Read the model definition and answer for the solid it produces. Units are mm, in the model's axes. Coordinates: 2 decimals unless noted, no trailing zeros. Order: outer loops, then holes, each group sorted by start corner. A loop starts at its lowest first (then second) coordinate and runs counter-clockwise, first axis right, second up. Notation, with made-up numbers: M 78.5,89 L 137.5,89 A25 cw 137.5,103 Z; hole C 69,-24 d11. An arc over 180 degrees is marked long. Write each question's results on one line, items separated by ' | '.
```python
from build123d import *

# Parameters (mm, degrees)
SKETCH12_R                   = 30.1625
SKETCH12_R_2                 = 26.2509
PIPE_STANDARD_S40_P2_1_DEPTH = 660.4
CUT_EXTRUDE1_DEPTH           = 662.7761803
CUT_EXTRUDE1_DEPTH_BACK      = 662.7761803
CUT_EXTRUDE2_DEPTH           = 662.7761803
CUT_EXTRUDE2_DEPTH_BACK      = 662.7761803
CUT_EXTRUDE3_DEPTH           = 662.7761803
CUT_EXTRUDE3_DEPTH_BACK      = 662.7761803


with BuildPart() as part:
    # Sketch12 → Pipe (standard, s40) P2(1) (new body)
    with BuildSketch(Plane(origin=(0, 0, 0), x_dir=(-1, 0, 0), z_dir=(0, 0, -1))):
        Circle(SKETCH12_R)
        Circle(SKETCH12_R_2, mode=Mode.SUBTRACT)
    extrude(amount=PIPE_STANDARD_S40_P2_1_DEPTH)

    # Sketch14 → Cut-Extrude1 (cut, two sides)
    with BuildSketch(Plane(origin=(0, 0, 0), x_dir=(1, 0, 0), z_dir=(0, 1, 0))) as cut_extrude1_sk:
        Polygon((0, 12.7), (-12.7, 0), (12.7, 0), align=None)
    extrude(amount=CUT_EXTRUDE1_DEPTH, mode=Mode.SUBTRACT)
    extrude(cut_extrude1_sk.sketch, amount=-CUT_EXTRUDE1_DEPTH_BACK, mode=Mode.SUBTRACT)

    # Sketch15 → Cut-Extrude2 (cut, two sides)
    with BuildSketch(Plane(origin=(0, 0, 0), x_dir=(0, 0, -1), z_dir=(0.8660254037844364, -0.5000000000000041, 0))) as cut_extrude2_sk:
        Polygon((0, 12.7), (0, -12.7), (12.7, 0), align=None)
    extrude(amount=CUT_EXTRUDE2_DEPTH, mode=Mode.SUBTRACT)
    extrude(cut_extrude2_sk.sketch, amount=-CUT_EXTRUDE2_DEPTH_BACK, mode=Mode.SUBTRACT)

    # Sketch16 → Cut-Extrude3 (cut, two sides)
    with BuildSketch(Plane(origin=(0, 0, 0), x_dir=(0, 0, -1), z_dir=(-0.8660254037844433, -0.49999999999999195, 0))) as cut_extrude3_sk:
        Polygon((0, 12.7), (0, -12.7), (12.7, 0), align=None)
    extrude(amount=CUT_EXTRUDE3_DEPTH, mode=Mode.SUBTRACT)
    extrude(cut_extrude3_sk.sketch, amount=-CUT_EXTRUDE3_DEPTH_BACK, mode=Mode.SUBTRACT)


solid = part.part
```
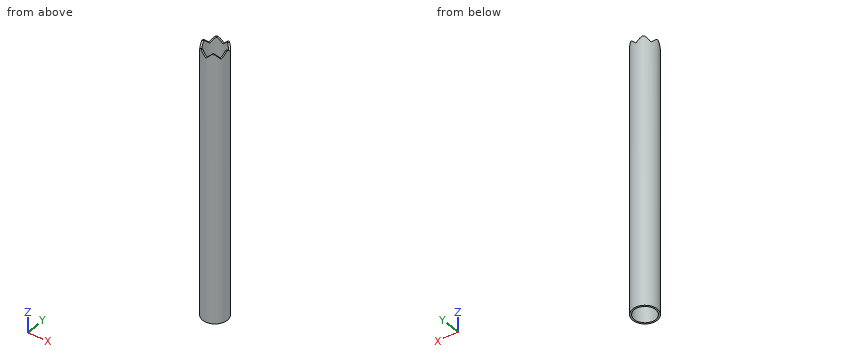
(1) Straight lines are drawn through the part: line 1 (Y direction, x = 0, z = -319); line 2 (Y direction, x = -22, z = -120.5); line 3 (X direction, y = -9.5, z = -580.5). For each, find the intervals that lie inside material, in ascending order.
Conclusion:
line 1: -30.16 to -26.25, 26.25 to 30.16 | line 2: -20.63 to -14.32, 14.32 to 20.63 | line 3: -28.63 to -24.47, 24.47 to 28.63
(2) The part is cut by section A-A, the plane z = -200. Write down the section's boundary in (x, y) (1 decimal).
Conclusion:
outline: C 0,0 d60.3; hole C 0,0 d52.5
(3) Given pin 1 (6 mm diameter, centred on x = 18.5, z = -212.5, fed in from -Y); pin 2 (12 mm diameter, centred on y = -9.5, z = -409.5, fed in from +X); pin 3 (12 mm diameter, centred on x = 8, z = -233.5, fed in from -Y), each flat-ended and moving along its own axis, determine where each tip first touches the part or whether it passes through.
Conclusion:
pin 1: y = -25.88 | pin 2: x = 29.96 | pin 3: y = -30.1
